```python
from build123d import *

# Parameters (mm, degrees)
F0_W     = 2
F0_H     = 12.7
F1_DEPTH = 12.7
F2_SIZE  = 0.635
F3_W     = 2.032
F3_H     = 5.08
F4_DEPTH = 25.4
F5_SIZE  = 1.01599


# Not quite as in the source:
# - a fillet or chamfer is up to 0.001 mm smaller than in the source, because OpenCascade refuses the exact size


with BuildPart() as f1:
    # F0 (on Top) → F1 (new body)
    with BuildSketch(Plane.XY):
        with BuildLine():
            Line((-15.1, -6.35), (-15.1, 6.35))
            Line((-15.1, 6.35), (-28.34, 6.35))
            ThreePointArc((-28.34, 6.35), (-26.7817380481, 3.3434490418), (-26.2442648116, 0))
            ThreePointArc((-26.2442648116, 0), (-26.7817380481, -3.3434490418), (-28.34, -6.35))
            Line((-28.34, -6.35), (-15.1, -6.35))
        make_face()
        with Locations((-14.1, 0)):
            Rectangle(F0_W, F0_H)
        with BuildLine():
            ThreePointArc((7.19, 13.1), (11.3690010768, 11.3690010768), (13.1, 7.19))
            Line((13.1, 7.19), (13.1, -7.19))
            ThreePointArc((13.1, -7.19), (11.3690010768, -11.3690010768), (7.19, -13.1))
            Line((7.19, -13.1), (-7.19, -13.1))
            ThreePointArc((-7.19, -13.1), (-11.3690010768, -11.3690010768), (-13.1, -7.19))
            Line((-13.1, -7.19), (-13.1, -6.35))
            Line((-13.1, -6.35), (-15.1, -6.35))
            Line((-15.1, -6.35), (-15.1, -7.19))
            ThreePointArc((-15.1, -7.19), (-12.7832146392, -12.7832146392), (-7.19, -15.1))
            Line((-7.19, -15.1), (7.19, -15.1))
            ThreePointArc((7.19, -15.1), (12.7832146392, -12.7832146392), (15.1, -7.19))
            Line((15.1, -7.19), (15.1, 7.19))
            ThreePointArc((15.1, 7.19), (12.7832146392, 12.7832146392), (7.19, 15.1))
            Line((7.19, 15.1), (-7.19, 15.1))
            ThreePointArc((-7.19, 15.1), (-12.7832146392, 12.7832146392), (-15.1, 7.19))
            Line((-15.1, 7.19), (-15.1, 6.35))
            Line((-15.1, 6.35), (-13.1, 6.35))
            Line((-13.1, 6.35), (-13.1, 7.19))
            ThreePointArc((-13.1, 7.19), (-11.3690010768, 11.3690010768), (-7.19, 13.1))
            Line((-7.19, 13.1), (7.19, 13.1))
        make_face()
    extrude(amount=F1_DEPTH)

    # F2
    f2_edges = [f1.edges().sort_by_distance(p)[0] for p in [
        (-11.369001, 11.369001, 12.7),
        (0, 13.1, 12.7),
        (11.369001, 11.369001, 12.7),
        (13.1, 0, 12.7),
        (11.369001, -11.369001, 12.7),
        (0, -13.1, 12.7),
        (-11.369001, -11.369001, 12.7),
        (-13.1, 0, 12.7),
    ]]
    chamfer(f2_edges, length=F2_SIZE)

    # F3 (on face) → F4 (cut)
    with BuildSketch(Plane.XZ.offset(6.35)):
        with Locations((-21.72, 6.35)):
            Rectangle(F3_W, F3_H)
    extrude(amount=-F4_DEPTH, mode=Mode.SUBTRACT)

    # F5 (size 1.016 in the source; OpenCascade refuses exactly that, so slightly less here)
    f5_edges = [f1.edges().sort_by_distance(p)[0] for p in [
        (-22.736, 0, 3.81),
        (-20.704, 0, 3.81),
        (-20.704, 0, 8.89),
        (-22.736, 0, 8.89),
    ]]
    chamfer(f5_edges, length=F5_SIZE)


solid = f1.part
```
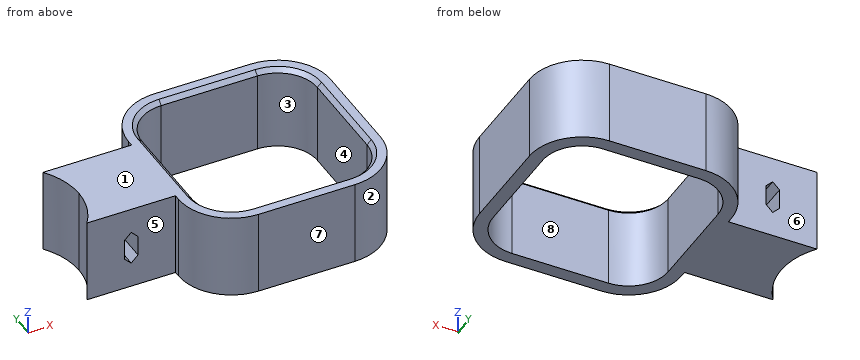
For this review, take the finished solid that the model builds, in its own axes (mm). Face numbers are marked on the shaded views. A direction names the side the tool comes from. Coordinates: 2 decimals unless noted, no trailing zeros. Loops run counter-clockwise (first coordinate to the right, second up) from the corner with the lowest first, then second, coordinate; pieces in that order, holes last.
1. Add section B-B, the plane x = 4.5. Give the boundary of the cut face in (y, z) (3 decimals).
2. For line 1 (Y direction, x = 1, z = 11.25); line 2 (Y direction, x = -21, z = 12.25), list the stretches that pass through material, from the lowest coordinate up.
3. Insertion check: P1, Ø6, axis at y = -3, z = 3, coming from the -X side; P2, Ø4, axis at x = -10, z = 8.5, coming from the -Y side; P3, Ø0.9, axis at y = 6.5, z = 3.5, coming from the -X side. Each pin has a flat end and moves straight along its axis. Give the tip position at first contact, or say it passes through.
4. Add section A-A, the plane z = 5.5. Give the boundary of the cut face in (x, y), then the cut area to 3 significant figures.
5. For the marked faces 5, 6, 7 and 8, list the 3-axis set-ups (+Z, -Z, +X, -X, +Y, -Y) from which the entire face can be reached by the end or side of a thin tool; tool diameter is ignored.
6. Mouldability with a two-part tool opening along X and no side actions: class the marked faces 1, 2, 3 and 4 as +X half, -X half, draft (parallel to the pull), parting line (faces both ways), or undercut.
7. Add section C-C, the plane y = -5.5. Count the separate pieces of the cut face and the enclosed holes in it, then the cut area to 3 significant figures.
8. Add section D-D, the plane z = 1.25. Give the boundary of the cut face in (x, y).
Result:
1. outline: (-15.1, 0) - (-13.1, 0) - (-13.1, 12.065) - (-13.735, 12.7) - (-15.1, 12.7) - close; (13.1, 0) - (15.1, 0) - (15.1, 12.7) - (13.735, 12.7) - (13.1, 12.065) - close
2. line 1: y = -15.1 to -13.1, 13.1 to 15.1
2. line 2: y = -6.35 to 6.35
3. P1: stops at x = -28.09
3. P2: stops at y = -15.06
3. P3: stops at x = -28.34
4. outline: (-28.34, -6.35) - (-22.74, -6.35) - (-22.74, 6.35) - (-28.34, 6.35) arc R10.67 cw to start; (-20.7, -6.35) - (-15.1, -6.35) - (-15.1, -7.19) arc R7.91 ccw to (-7.19, -15.1) - (7.19, -15.1) arc R7.91 ccw to (15.1, -7.19) - (15.1, 7.19) arc R7.91 ccw to (7.19, 15.1) - (-7.19, 15.1) arc R7.91 ccw to (-15.1, 7.19) - (-15.1, 6.35) - (-20.7, 6.35) - close; hole (-13.1, -7.19) arc R5.91 ccw to (-7.19, -13.1) - (7.19, -13.1) arc R5.91 ccw to (13.1, -7.19) - (13.1, 7.19) arc R5.91 ccw to (7.19, 13.1) - (-7.19, 13.1) arc R5.91 ccw to (-13.1, 7.19) - close
4. area: 326 mm2
5. face 5: +Z, -Z, -X, -Y
5. face 6: +Z, -Z, -X, +Y
5. face 7: +Z, -Z, +X, -X, -Y
5. face 8: +Z, -Z
6. face 1: draft
6. face 2: +X half
6. face 3: undercut
6. face 4: undercut
7. separate pieces: 2
7. enclosed holes: 1
7. area: 203 mm2
8. outline: (-28.34, -6.35) - (-15.1, -6.35) - (-15.1, -7.19) arc R7.91 ccw to (-7.19, -15.1) - (7.19, -15.1) arc R7.91 ccw to (15.1, -7.19) - (15.1, 7.19) arc R7.91 ccw to (7.19, 15.1) - (-7.19, 15.1) arc R7.91 ccw to (-15.1, 7.19) - (-15.1, 6.35) - (-28.34, 6.35) arc R10.67 cw to start; hole (-13.1, -7.19) arc R5.91 ccw to (-7.19, -13.1) - (7.19, -13.1) arc R5.91 ccw to (13.1, -7.19) - (13.1, 7.19) arc R5.91 ccw to (7.19, 13.1) - (-7.19, 13.1) arc R5.91 ccw to (-13.1, 7.19) - close
